```python
from build123d import *

# Parameters (mm, degrees)
SKETCH1_R           = 2.025
SKETCH1_R_2         = 1.2295
BOSS_EXTRUDE1_DEPTH = 4
BOSS_EXTRUDE3_START = 29.25
BOSS_EXTRUDE3_DEPTH = 29.25


with BuildPart() as part:
    # Sketch1 → Boss-Extrude1 (new body)
    with BuildSketch(Plane.YZ):
        with BuildLine():
            Line((-11.385441559, -10.385441559), (-5.828427125, -4.828427125))
            ThreePointArc((-5.828427125, -4.828427125), (-3.73508426, -1.69551813), (-3, 2))
            Line((-3, 2), (-3, 8))
            ThreePointArc((-3, 8), (2, 13), (7, 8))
            Line((7, 8), (7, 4.071067812))
            ThreePointArc((7, 4.071067812), (6.619397663, 2.15765065), (5.535533906, 0.535533906))
            Line((5.535533906, 0.535533906), (-1, -6))
            Line((-1, -6), (-1, -11))
            Line((-1, -11), (-11.130883118, -11))
            ThreePointArc((-11.130883118, -11), (-11.463479749, -10.777766036), (-11.385441559, -10.385441559))
        make_face()
        with Locations(Location((2, 8, 0), (0, 0, 270))):
            Circle(SKETCH1_R, mode=Mode.SUBTRACT)
        with Locations(Location((0, 0, 0), (0, 0, 270))):
            Circle(SKETCH1_R_2, mode=Mode.SUBTRACT)
    boss_extrude1 = extrude(amount=BOSS_EXTRUDE1_DEPTH)

    # Sketch4 → Boss-Extrude3 (add)
    with BuildSketch(Plane(origin=(0, 0, 0), x_dir=(0, -1, 0), z_dir=(-1, 0, 0)).offset(BOSS_EXTRUDE3_START)):
        with BuildLine():
            Line((1, -6), (1, -11))
            Line((1, -11), (11.130883118, -11))
            ThreePointArc((11.130883118, -11), (11.463479749, -10.777766036), (11.385441559, -10.385441559))
            Line((11.385441559, -10.385441559), (7, -6))
            Line((7, -6), (6, -5))
            Line((6, -5), (1, -5))
            Line((1, -5), (1, -6))
        make_face()
    boss_extrude3 = extrude(amount=-BOSS_EXTRUDE3_DEPTH)

    # Mirror8: Boss-Extrude3 across plane
    add(boss_extrude3.mirror(Plane(origin=(-29.25, 0, 0), x_dir=(0, 0, 1), z_dir=(1, 0, 0))))

    # Mirror9: Boss-Extrude1 across plane
    add(boss_extrude1.mirror(Plane(origin=(-29.25, 0, 0), x_dir=(0, 0, 1), z_dir=(1, 0, 0))))


solid = part.part
```
Design review of the part built by this model. Coordinates are the model's own, in mm. A direction names the side the tool comes from. Round coordinates to 2 decimals unless told otherwise and drop trailing zeros. Write each loop counter-clockwise with the first axis right and the second up, starting at its lowest first coordinate (ties: lowest second). Pieces come first, ordered by that corner, then holes. Notation, with made-up numbers: (-36.5, 78.25) -> (20.5, 78.25) arc R10 ccw to (20.5, 92.25) -> close; hole circle Ø3 at (33, 50.5). An arc over 180 degrees is marked (long way). Answer in a Markdown table with one row per item.
Q1. Take a section at B-B, the plane x = -55.5. State the section outline as (y, z) points.
The answers:
| item | result |
|---|---|
| outline | (-11.39, -10.39) arc R0.36 ccw to (-11.13, -11) -> (-1, -11) -> (-1, -5) -> (-6, -5) -> close |
Q2. Take a section at D-D, the plane y = -7.5. State the section outline as (x, z) points, then the cut area to 3 significant figures.
The answers:
| item | result |
|---|---|
| outline | (-62.5, -11) -> (4, -11) -> (4, -6.5) -> (-62.5, -6.5) -> close |
| area | 299 mm² |
Q3. Take a section at A-A, the plane y = 2. State the section outline as (x, z) points (3 decimals).
The answers:
| item | result |
|---|---|
| outline | (-62.5, -3) -> (-58.5, -3) -> (-58.5, 5.975) -> (-62.5, 5.975) -> close; (-62.5, 10.025) -> (-58.5, 10.025) -> (-58.5, 13) -> (-62.5, 13) -> close; (0, -3) -> (4, -3) -> (4, 5.975) -> (0, 5.975) -> close; (0, 10.025) -> (4, 10.025) -> (4, 13) -> (0, 13) -> close |
Q4. Take a section at C-C, the plane z = -8.75. State the section outline as (x, y) points.
The answers:
| item | result |
|---|---|
| outline | (-62.5, -9.75) -> (4, -9.75) -> (4, -1) -> (-62.5, -1) -> close |
Q5. Draft analysis for pull direction X (two halves, no side actions). For faces 4 (the face through (0, 1, 4)), 5 (the face through (4, -2, 1)), 6 (the face through (2, -3, 5)), state which applies: +X half, -X half, draft (parallel to the pull), parting line (faces both ways), or undercut.
The answers:
| item | result |
|---|---|
| face 4 | undercut |
| face 5 | +X half |
| face 6 | draft |
Q6. Clearance check with flat-ended pins moving along their axes: pin 1 Ø3.5 at (y, z) = (2, 8) entering from -X; pin 2 Ø3 at (x, z) = (-60.5, 6.5) entering from -Y; pin 3 Ø5 at (x, y) = (-46.5, -9) entering from +Z; pin 4 Ø1 at (x, y) = (-13.5, -8.5) entering from +Z. State where each tip first meets the part, or that it passes through.
The answers:
| item | result |
|---|---|
| pin 1 | through |
| pin 2 | y = -3 |
| pin 3 | z = -5.5 |
| pin 4 | z = -7 |
Q7. For faces 1 (the face through (-60.47, 6.63, 2.18)), 2 (the face through (-29, -4, -5)), 3 (the face through (-60, -3, 5)), list the 3-axis set-ups (+Z, -Z, +X, -X, +Y, -Y) from which the entire face can be reached by the end or side of a thin tool; tool diameter is ignored.
The answers:
| item | result |
|---|---|
| face 1 | -Z, +X, -X, +Y |
| face 2 | +Z, +Y, -Y |
| face 3 | +Z, +X, -X, -Y |
Q8. To check wall thickness, follow L1, parallel to X at y = 3.5, z = 5; L2, parallel to Z at x = -24.5, y = -5.5; L3, parallel to Y at x = -60.45, z = 0. State the ranges of each line that lie inside material, in increasing order. Write a range as [from, to].
The answers:
| item | result |
|---|---|
| L1 | [-62.5, -58.5], [0, 4] |
| L2 | [-11, -5] |
| L3 | [-3.21, -1.23], [1.23, 5] |
